Geometry: final body of the model. Coordinates: model frame, mm. A direction names the side the tool comes from. Round coordinates to 2 decimals unless told otherwise and drop trailing zeros. Loops run counter-clockwise (first coordinate to the right, second up) from the corner with the lowest first, then second, coordinate; pieces in that order, holes last. Notation, with made-up numbers: (5, 8) - (11, 8) arc R21 ccw to (11, 16) - close; hole circle Ø1 at (-31.75, -7). An arc over 180 degrees is marked (long way). Write item = value, one per line. Start each with the question number.
Item 1: Section A-A (y = -4). Return loops of the section in (x, z).
Item 2: Draft query along X for faces 3 (the flat face through (5, -2, 5)), 4 (the flat face through (8, -8.01, 1)), 5 (the cylindrical face through (-0.552, -0.986, 7.294)). Return one class per face: pulls with the +X half, pulls with the -X half, needs draft (parallel to the pull), parting line crosses it, or undercut.
Item 3: First-contact query: pin 1 (1.2 mm diameter, centred on x = 2.5, z = 6, fed in from -Y); pin 2 (3 mm diameter, centred on x = -1.5, z = -4, fed in from -Y); pin 3 (2.5 mm diameter, centred on x = 3.5, z = 4.5, fed in from -Y); pin 4 (5.5 mm diameter, centred on x = 0, z = 0, fed in from +Y). Flat tips, straight axial feed; report the tip coordinate or a pass-through.
Item 4: Line query: line 1 (X direction, y = -2.75, z = 2.25); line 2 (X direction, y = -1, z = 1.25); line 3 (Y direction, x = -8.5, z = 1.25). Output: solid intervals per line, ascending. Write a range as from..to.
Item 5: Access query for faces 1 (the cylindrical face through (1.113, 0.993, 7.799)), 2 (the cylindrical face through (4.373, -0.986, 5.981)). Directions: +Z, -Z, +X, -X, +Y, -Y. A direction counts if a zero-diameter tool reaches every point of the face in a straight line with its end or side. Return the directions, or none.
from build123d import *
from build123d.topology import SkipClean

# Parameters (mm, degrees)
SKETCH1_R                                       = 9.5
BOSS_EXTRUDE1_DEPTH                             = 1.5
SKETCH2_R                                       = 4.5
CUT_EXTRUDE1_DEPTH                              = 14.518505835
SKETCH3_R                                       = 2
CUT_EXTRUDE5_DEPTH                              = 0.5
SKETCH4_R                                       = 1.35
CUT_EXTRUDE6_DEPTH                              = 14.518505835
BOSS_EXTRUDE2_DEPTH                             = 2
CIRPATTERN1_OUTLINE_R                           = 1.35
CIRPATTERN1_DEPTH                               = 1.5
CIRPATTERN1_2_OUTLINE_R                         = 2
CIRPATTERN1_2_OUTLINE_R_2                       = 1.35
CIRPATTERN1_2_DEPTH                             = 0.5
BOSS_EXTRUDE3_DEPTH                             = 6.01
CSK_FOR_M2_FLAT_HEAD_MACHINE_SCREW1_D           = 2.2
CSK_FOR_M2_FLAT_HEAD_MACHINE_SCREW1_CSINK_D     = 4.4
CSK_FOR_M2_FLAT_HEAD_MACHINE_SCREW1_CSINK_ANGLE = 90


# Read off the part's stored shape, not the designer's step: CirPattern1, CirPattern2
with BuildPart() as part:
    # Sketch1 → Boss-Extrude1 (new body)
    with BuildSketch(Plane(origin=(0, 0, 0), x_dir=(1, 0, 0), z_dir=(0, 1, 0))):
        with Locations(Location((0, 0, 0), (0, 0, 270))):
            Circle(SKETCH1_R)
    extrude(amount=BOSS_EXTRUDE1_DEPTH)

    # Sketch2 → Cut-Extrude1 (cut, through all)
    with BuildSketch(Plane(origin=(0, 1.5, 0), x_dir=(1, 0, 0), z_dir=(0, 1, 0))):
        with Locations(Location((0, 0, 0), (0, 0, 270))):
            Circle(SKETCH2_R)
    extrude(amount=-CUT_EXTRUDE1_DEPTH, mode=Mode.SUBTRACT)

    # Sketch3 → Cut-Extrude5 (cut)
    with BuildSketch(Plane.XZ):
        with Locations(Location((1.93443789, 6.72740292, 0), (0, 0, 270))):
            Circle(SKETCH3_R)
    extrude(amount=-CUT_EXTRUDE5_DEPTH, mode=Mode.SUBTRACT)

    # Sketch4 → Cut-Extrude6 (cut, through all)
    with BuildSketch(Plane.XZ):
        with Locations(Location((1.93443789, 6.72740292, 0), (0, 0, 270))):
            Circle(SKETCH4_R)
    extrude(amount=-CUT_EXTRUDE6_DEPTH, mode=Mode.SUBTRACT)

    # Sketch5 → Boss-Extrude2 (add)
    with SkipClean():  # the faces are left unmerged after this step: merging them gives an invalid solid
        with BuildSketch(Plane.XZ):
            with BuildLine():
                ThreePointArc((3.182648464, 8.951019425), (4.357780459, 5.933733723), (1.625396676, 4.196198952))
                ThreePointArc((1.625396676, 4.196198952), (4.436036831, 0.756027269), (2.92357195, -3.420924883))
                ThreePointArc((2.92357195, -3.420924883), (6.077241126, -4.155308257), (5.967881507, -7.391507987))
                ThreePointArc((5.967881507, -7.391507987), (9.364966644, 1.596057567), (3.182648464, 8.951019425))
            make_face()
            with BuildLine():
                ThreePointArc((0.851769477, 4.418652369), (-0.540347051, 7.342170761), (2.058000389, 9.274407496))
                ThreePointArc((2.058000389, 9.274407496), (-7.086809251, 6.326700138), (-8.982537647, -3.092574561))
                ThreePointArc((-8.982537647, -3.092574561), (-7.356211508, -0.292572507), (-4.294138699, -1.34550096))
                ThreePointArc((-4.294138699, -1.34550096), (-3.356909645, 2.99685796), (0.851769477, 4.418652369))
            make_face()
            with BuildLine():
                ThreePointArc((-8.534166016, -4.173488997), (-2.625308565, -9.13004682), (5.013839927, -8.069164095))
                ThreePointArc((5.013839927, -8.069164095), (1.922148158, -7.106672419), (2.267302196, -3.887073546))
                ThreePointArc((2.267302196, -3.887073546), (-1.243567215, -4.32475902), (-3.985711115, -2.089044497))
                ThreePointArc((-3.985711115, -2.089044497), (-5.403439375, -5.000228929), (-8.534166016, -4.173488997))
            make_face()
        extrude(amount=BOSS_EXTRUDE2_DEPTH)

    # CirPattern1 outline → CirPattern1 (cut)
    with SkipClean():  # the faces are left unmerged after this step: merging them gives an invalid solid
        with BuildSketch(Plane(origin=(0, 0, 0), x_dir=(1, 0, 0), z_dir=(0, 1, 0))):
            with Locations((4.053593102, 5.706871557)):
                Circle(CIRPATTERN1_OUTLINE_R)
            with Locations((-6.465797695, 2.68206267)):
                Circle(CIRPATTERN1_OUTLINE_R)
        extrude(amount=CIRPATTERN1_DEPTH, mode=Mode.SUBTRACT)

    # CirPattern1 2 outline → CirPattern1 2 (cut)
    # profile 1 of 2: a face of its own
    with SkipClean():  # the faces are left unmerged after this step: merging them gives an invalid solid
        with BuildSketch(Plane(origin=(0, 0, 0), x_dir=(1, 0, 0), z_dir=(0, 1, 0))):
            with Locations((-6.465797695, 2.68206267)):
                Circle(CIRPATTERN1_2_OUTLINE_R)
            with Locations((-6.465797695, 2.68206267)):
                Circle(CIRPATTERN1_2_OUTLINE_R_2, mode=Mode.SUBTRACT)
        # profile 2 of 2: a face of its own
        with BuildSketch(Plane(origin=(0, 0, 0), x_dir=(1, 0, 0), z_dir=(0, 1, 0))):
            with Locations((4.053593102, 5.706871557)):
                Circle(CIRPATTERN1_2_OUTLINE_R)
            with Locations((4.053593102, 5.706871557)):
                Circle(CIRPATTERN1_2_OUTLINE_R_2, mode=Mode.SUBTRACT)
        extrude(amount=CIRPATTERN1_2_DEPTH, mode=Mode.SUBTRACT)

    # Sketch9 → Boss-Extrude3 (add)
    with SkipClean():  # the faces are left unmerged after this step: merging them gives an invalid solid
        with BuildSketch(Plane.XZ.offset(2)):
            with BuildLine():
                ThreePointArc((-9.476901231, 0.662074811), (-6.993614762, 1.786875586), (-4.31661582, 1.271545462))
                ThreePointArc((-4.31661582, 1.271545462), (-3.356909645, 2.99685796), (-1.751062326, 4.145332403))
                ThreePointArc((-1.751062326, 4.145332403), (-2.565519544, 6.746975713), (-1.728461612, 9.341435674))
                ThreePointArc((-1.728461612, 9.341435674), (-7.086809251, 6.326700138), (-9.476901231, 0.662074811))
            make_face()
            with BuildLine():
                ThreePointArc((6.426382202, 6.996542846), (5.757483071, 4.353729492), (3.685500216, 2.582070517))
                ThreePointArc((3.685500216, 2.582070517), (4.436036831, 0.756027269), (4.332720881, -1.215536824))
                ThreePointArc((4.332720881, -1.215536824), (6.874573296, -2.200866602), (8.38110669, -4.472924173))
                ThreePointArc((8.38110669, -4.472924173), (9.364966644, 1.596057567), (6.426382202, 6.996542846))
            make_face()
            with BuildLine():
                ThreePointArc((1.4633337, -9.386621036), (-0.185849196, -7.215887463), (-0.279127779, -4.491334733))
                ThreePointArc((-0.279127779, -4.491334733), (-1.243567215, -4.32475902), (-2.149181875, -3.953608133))
                ThreePointArc((-2.149181875, -3.953608133), (-3.675422752, -6.212474499), (-6.225750314, -7.175655582))
                ThreePointArc((-6.225750314, -7.175655582), (-2.625308565, -9.13004682), (1.4633337, -9.386621036))
            make_face()
        extrude(amount=BOSS_EXTRUDE3_DEPTH)

    # CSK for M2 Flat Head Machine Screw1 (through all)
    with Locations(Plane(origin=(0, 1.5, 0), x_dir=(1, 0, 0), z_dir=(0, 1, 0))):
        with Locations((-1.93443789, 6.72740292)):
            CounterSinkHole(CSK_FOR_M2_FLAT_HEAD_MACHINE_SCREW1_D / 2, CSK_FOR_M2_FLAT_HEAD_MACHINE_SCREW1_CSINK_D / 2, counter_sink_angle=CSK_FOR_M2_FLAT_HEAD_MACHINE_SCREW1_CSINK_ANGLE)

    # CirPattern2 outline → CirPattern2 (revolve, cut)
    with SkipClean():  # the faces are left unmerged after this step: merging them gives an invalid solid
        with BuildSketch(Plane(origin=(6.793320775, 0, 1.688429105), x_dir=(1, 0, 0), z_dir=(0, 0, 1))):
            Polygon((0, -8.01), (1.1, -8.01), (1.1, 0.4), (2.2, 1.5), (0, 1.5), align=None)
        revolve(axis=Axis((6.793320775, 0, 1.688429105), (0, 1, 0)), mode=Mode.SUBTRACT)

    # CirPattern2 2 outline → CirPattern2 2 (revolve, cut)
    with SkipClean():  # the faces are left unmerged after this step: merging them gives an invalid solid
        with BuildSketch(Plane(origin=(-4.858882885, 0, 5.038973815), x_dir=(1, 0, 0), z_dir=(0, 0, 1))):
            Polygon((0, -8.01), (1.1, -8.01), (1.1, 0.4), (2.2, 1.5), (0, 1.5), align=None)
        revolve(axis=Axis((-4.858882885, 0, 5.038973815), (0, 1, 0)), mode=Mode.SUBTRACT)


solid = part.part
Taken from the geometry:
q1.outline = (-9.48, 0.66) arc R4.5 cw to (-4.32, 1.27) arc R4.5 cw to (-1.75, 4.15) arc R4.5 cw to (-1.73, 9.34) arc R9.5 ccw to start; (-6.23, -7.18) arc R9.5 ccw to (1.46, -9.39) arc R4.5 cw to (-0.28, -4.49) arc R4.5 cw to (-2.15, -3.95) arc R4.5 cw to start; (3.69, 2.58) arc R4.5 cw to (4.33, -1.22) arc R4.5 cw to (8.38, -4.47) arc R9.5 ccw to (6.43, 7) arc R4.5 cw to start; hole circle Ø2.2 at (-4.86, 5.04); hole circle Ø2.2 at (-1.93, -6.73); hole circle Ø2.2 at (6.79, 1.69)
q2.face_3 = undercut
q2.face_4 = needs draft
q2.face_5 = undercut
q3.pin_1 = 0.5
q3.pin_2 = -8.01
q3.pin_3 = -2
q3.pin_4 = through
q4.line_1 = -9.23..-3.9, 3.9..5.85, 7.74..9.23
q4.line_2 = -9.42..-4.32, 4.32..5.78, 7.8..9.42
q4.line_3 = -2..1.5
q5.face_1 = +Y, -Y
q5.face_2 = -Y
